CAD build for the part. Positions are in the model's coordinates, mm. Face numbers are marked on the shaded views. A direction names the side the tool comes from. Coordinates: 2 decimals unless noted, no trailing zeros. Write each loop counter-clockwise with the first axis right and the second up, starting at its lowest first coordinate (ties: lowest second). Pieces come first, ordered by that corner, then holes. Notation, with made-up numbers: (42.25, -8.5) -> (87.25, -8.5) arc R13 ccw to (87.25, -0.5) -> close; hole circle Ø8 at (60.25, 55). An arc over 180 degrees is marked (long way). Answer as CSV lines item,"result".
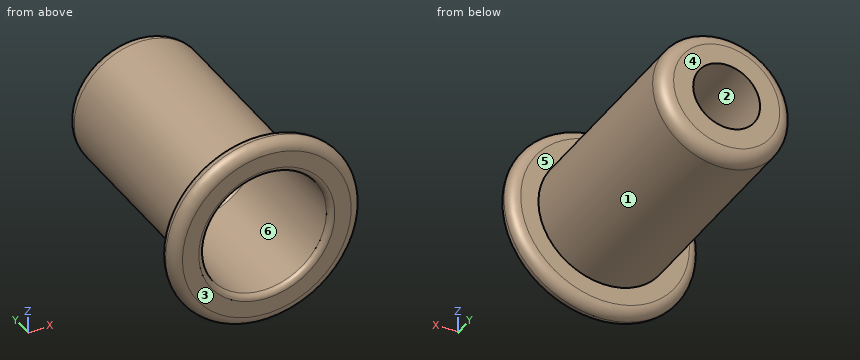
Autodesk Inventor part; units mm, degrees
ref_plane "YZ Plane" through (0, 0, 0) normal (1, 0, 0) x (0, 1, 0)
ref_plane "XZ Plane" through (0, 0, 0) normal (0, 1, 0) x (-1, 0, 0)
ref_plane "XY Plane" through (0, 0, 0) normal (0, 0, 1) x (1, 0, 0)
sketch "スケッチ1" plane through (0, 0, 0) normal (0, 1, 0) x (-1, 0, 0)
  circle A0 centre (0, 0) radius 3.5
  dimension "d0" = 7
extrude "押し出し1" add sketch "スケッチ1" along normal blind 0.8
sketch "スケッチ2" plane through (0, 0.8, 0) normal (0, 1, 0) x (1, 0, 0)
  circle A0 centre (0, 0) radius 2.45
  dimension "d3" = 4.9
extrude "押し出し2" add sketch "スケッチ2" along normal blind 8.2
fillet "フィレット1" radius 0.4 2 edges at (3.5, 0, 0) (3.5, 0.8, 0)
sketch "スケッチ3" plane through (0, 0, 0) normal (0, -1, 0) x (1, 0, 0)
  point P0 (0, 0)
  point P1 (0, 0)
hole "穴1" at (0, 0, 0) direction (0, 1, 0) diameter 2.459 end through all counterbore diameter 4.6 counterbore depth 5
fillet "フィレット2" radius 0.2 2 edges at (0, 0, 2.3) (0, 5, 2.3)
fillet "フィレット2" radius 0.5 1 edges at (-2.45, 9, 0)
properties part number "M3-RivetNut"
Item 1: Flat gauge pins, fed straight in: pin 1 (3 mm diameter, centred on x = 0, z = 0, fed in from -Y); pin 2 (1 mm diameter, centred on y = 7, z = 2, fed in from -X); pin 3 (3 mm diameter, centred on x = 1.5, y = 4, fed in from -Z). Where does each tip first touch, or does it go through?
Answer below:
pin 1,"stops at y = 5"
pin 2,"stops at x = -1.94"
pin 3,"stops at z = -2.45"
Item 2: Saw through at D-D on y = 7.5. Give the cut face in (x, z), and give its area (3 significant figures).
Answer below:
outline,"circle Ø4.9 at (0, 0); hole circle Ø2.46 at (0, 0)"
area,"14.1 mm2"
Item 3: 3-axis set-ups, long thin cutter, end or side, ignore diameter. For the marked faces 4, 5 and 6: which of +Z, -Z, +X, -X, +Y, -Y reach the whole face in a straight line?
Answer below:
face 4,"+Z, -Z, +X, -X, +Y"
face 5,"+Y"
face 6,"-Y"
Item 4: Two-plate mould, pull along Z, no slides. Class the marked faces 1, 2 and 3: pulls with the +Z half, pulls with the -Z half, needs draft (parallel to the pull), parting line crosses it, or undercut.
Answer below:
face 1,"parting line crosses it"
face 2,"undercut"
face 3,"needs draft"
Item 5: Saw through at C-C on y = 2. Give the cut face in (x, z).
Answer below:
outline,"circle Ø4.9 at (0, 0); hole circle Ø4.6 at (0, 0)"
Item 6: Wall check: line 1 (X direction, y = 1.75, z = 0); line 2 (X direction, y = 8.2, z = 0). Give the ranges that are in metal, low to high. Write a range as from..to.
Answer below:
line 1,"x = -2.45..-2.3, 2.3..2.45"
line 2,"x = -2.45..-1.23, 1.23..2.45"
